Read the model definition and answer for the solid it produces. Units are mm, in the model's axes. Coordinates: 2 decimals unless noted, no trailing zeros. Loops run counter-clockwise (first coordinate to the right, second up) from the corner with the lowest first, then second, coordinate; pieces in that order, holes last. Notation, with made-up numbers: (84.5, 50.25) - (114.5, 50.25) arc R25 cw to (114.5, 67.25) - close; hole circle Ø1 at (-2.75, 52.25). An arc over 180 degrees is marked (long way). Use one line per item in the form item = value.
from build123d import *

# Parameters (mm, degrees)
SKETCH_1_R      = 1.6
SKETCH_1_R_2    = 5.5
EXTRUDE_1_DEPTH = 3


with BuildPart() as part:
    # 草图1 → 凸台-拉伸1 (new body)
    with BuildSketch(Plane(origin=(0, 0, 0), x_dir=(1, 0, 0), z_dir=(0, 1, 0))):
        Polygon((-46, 3), (-38, 11), (38, 11), (46, 3), (46, -3), (38, -11), (-38, -11), (-46, -3), align=None)
        with Locations(Location((0, 8, 0), (0, 0, 270))):
            Circle(SKETCH_1_R, mode=Mode.SUBTRACT)
        with Locations(Location((8, 0, 0), (0, 0, 270))):
            Circle(SKETCH_1_R, mode=Mode.SUBTRACT)
        with Locations(Location((-8, 0, 0), (0, 0, 90))):
            Circle(SKETCH_1_R, mode=Mode.SUBTRACT)
        with Locations(Location((0, 0, 0), (0, 0, 270))):
            Circle(SKETCH_1_R_2, mode=Mode.SUBTRACT)
        with Locations(Location((0, -8, 0), (0, 0, 90))):
            Circle(SKETCH_1_R, mode=Mode.SUBTRACT)
        with Locations(Location((-18, 0, 0), (0, 0, 270))):
            Circle(SKETCH_1_R, mode=Mode.SUBTRACT)
        with Locations(Location((-14, 5, 0), (0, 0, 270))):
            Circle(SKETCH_1_R, mode=Mode.SUBTRACT)
        with Locations(Location((-14, -5, 0), (0, 0, 90))):
            Circle(SKETCH_1_R, mode=Mode.SUBTRACT)
        with Locations(Location((14, -5, 0), (0, 0, 270))):
            Circle(SKETCH_1_R, mode=Mode.SUBTRACT)
        with Locations(Location((18, 0, 0), (0, 0, 90))):
            Circle(SKETCH_1_R, mode=Mode.SUBTRACT)
        with Locations(Location((14, 5, 0), (0, 0, 90))):
            Circle(SKETCH_1_R, mode=Mode.SUBTRACT)
        with Locations(Location((-41, 0, 0), (0, 0, 270))):
            Circle(SKETCH_1_R, mode=Mode.SUBTRACT)
        with Locations(Location((41, 0, 0), (0, 0, 90))):
            Circle(SKETCH_1_R, mode=Mode.SUBTRACT)
    extrude(amount=EXTRUDE_1_DEPTH)


solid = part.part
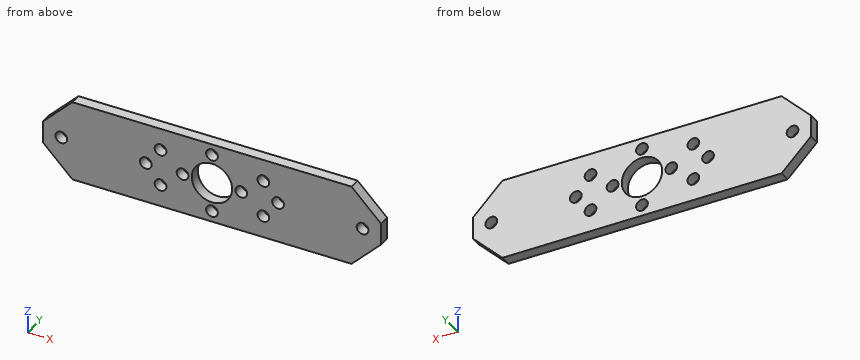
Item 1: The part is cut by section B-B on z = 0. Count the separate pieces of the cut face and the enclosed holes in it, plus the area to 3 significant figures.
Results below:
separate_pieces = 8
enclosed_holes = 0
area = 185 mm²
Item 2: The part is cut by section C-C on x = -14. Give the vertices of the cut face in (y, z).
Results below:
outline = (0, -11) - (3, -11) - (3, -6.6) - (0, -6.6) - close; (0, -3.4) - (3, -3.4) - (3, 3.4) - (0, 3.4) - close; (0, 6.6) - (3, 6.6) - (3, 11) - (0, 11) - close
Item 3: This flat-tipped pin is pushed along its axis until it touches: P1, Ø3.5, axis at x = 18, z = 0, coming from the -Y side. Where does it stop, or does it pass through?
Results below:
P1 = 0
Item 4: Find the intervals of material crossed by L1, parallel to X at y = 0.7, z = -6; L2, parallel to X at y = 0.95, z = -5.75; L3, parallel to X at y = 2.2, z = -5, in increasing order.
Results below:
L1 = -43 to -15.25, -12.75 to 12.75, 15.25 to 43
L2 = -43.25 to -15.41, -12.59 to 12.59, 15.41 to 43.25
L3 = -44 to -15.6, -12.4 to -2.29, 2.29 to 12.4, 15.6 to 44
Item 5: The part is cut by section A-A on x = 41. Give the vertices of the cut face in (y, z), plus the area to 3 significant figures.
Results below:
outline = (0, -8) - (3, -8) - (3, -1.6) - (0, -1.6) - close; (0, 1.6) - (3, 1.6) - (3, 8) - (0, 8) - close
area = 38.4 mm²
